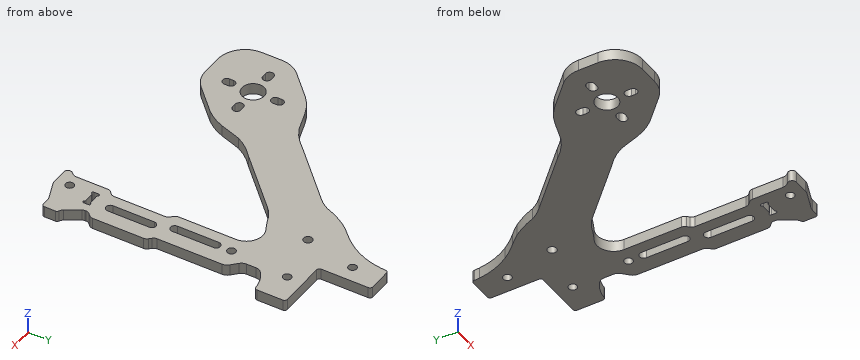
from build123d import *

# Parameters (mm, degrees)
F0_R     = 4
F0_R_2   = 1.5
F0_R_3   = 1.6
F1_DEPTH = 4


# Not quite as in the source:
# - ends of sketch curves that miss each other by under 0.0002 mm in the source are joined


with BuildPart() as f1:
    # F0 (on Top) → F1 (new body)
    with BuildSketch(Plane.XY):
        with BuildLine():
            ThreePointArc((30.9978440056, -52.3819660063), (30.5965854602, -54.0352331312), (31.997844, -55))
            Line((31.997844, -55), (37.420097, -55))
            ThreePointArc((37.420097, -55), (37.9874195635, -54.9458691602), (38.5342690291, -54.7854300727))
            Line((38.5342690291, -54.7854300727), (44.961419, -52.21457))
            ThreePointArc((44.961419, -52.21457), (45.5082684365, -52.0541308398), (46.075591, -52))
            Line((46.075591, -52), (48.497844, -52))
            ThreePointArc((48.497844, -52), (49.2049507812, -51.7071067812), (49.497844, -51))
            Line((49.497844, -51), (49.497844, -47.054858))
            ThreePointArc((49.497844, -47.054858), (49.3143367471, -46.477502309), (48.8311648121, -46.1120445316))
            ThreePointArc((48.8311648121, -46.1120445316), (48.2464480359, -45.7865652768), (47.8018474974, -45.2864046891))
            Line((47.8018474974, -45.2864046891), (44.801847, -40.486405))
            ThreePointArc((44.801847, -40.486405), (44.5753463762, -39.9777725676), (44.497844, -39.426408))
            Line((44.497844, -39.426408), (44.497844, -39.145707))
            ThreePointArc((44.497844, -39.145707), (44.650084935, -38.3803401353), (45.0836304376, -37.7314934376))
            Line((45.0836304376, -37.7314934376), (45.912058, -36.903066))
            ThreePointArc((45.912058, -36.903066), (46.3456032003, -36.2542195381), (46.497844, -35.488853))
            Line((46.497844, -35.488853), (46.497844, -17.145707))
            ThreePointArc((46.497844, -17.145707), (46.345603065, -16.3803401353), (45.9120575624, -15.7314934376))
            Line((45.9120575624, -15.7314934376), (45.08363, -14.903066))
            ThreePointArc((45.08363, -14.903066), (44.6500847997, -14.2542195381), (44.497844, -13.488853))
            Line((44.497844, -13.488853), (44.497844, 9.963987))
            ThreePointArc((44.497844, 9.963987), (44.2491834617, 11.1598679166), (43.5444232222, 12.1575032382))
            Line((43.5444232222, 12.1575032382), (41.451265, 14.110446))
            ThreePointArc((41.451265, 14.110446), (40.7465046743, 15.1080817706), (40.497844, 16.303963))
            Line((40.497844, 16.303963), (40.497844, 19.657184))
            ThreePointArc((40.497844, 19.657184), (40.8005276064, 20.970380205), (41.6475001819, 22.0185877679))
            ThreePointArc((41.6475001819, 22.0185877679), (44.9097367641, 23.8722057946), (48.5706879935, 24.6941080891))
            ThreePointArc((48.5706879935, 24.6941080891), (49.2302523646, 25.0105853837), (49.497844, 25.691451))
            Line((49.497844, 25.691451), (49.497844, 35))
            ThreePointArc((49.497844, 35), (49.2049507812, 35.7071067812), (48.497844, 36))
            Line((48.497844, 36), (31.497844, 36))
            ThreePointArc((31.497844, 36), (30.7907372188, 36.2928932188), (30.497844, 37))
            Line((30.497844, 37), (30.497844, 54))
            ThreePointArc((30.497844, 54), (30.2049507812, 54.7071067812), (29.497844, 55))
            Line((29.497844, 55), (21.513528, 55))
            ThreePointArc((21.513528, 55), (20.8178624993, 54.7183658616), (20.5140433064, 54.0320990223))
            ThreePointArc((20.5140433064, 54.0320990223), (20.4696724232, 53.1001685974), (20.3964907955, 52.1700570193))
            ThreePointArc((20.3964907955, 52.1700570193), (19.0508324444, 46.0085107955), (16.2674640132, 40.3491549914))
            ThreePointArc((16.2674640132, 40.3491549914), (14.1457607442, 37.4387671742), (11.7343381171, 34.7635058829))
            ThreePointArc((11.7343381171, 34.7635058829), (10.1184707238, 33.0449295675), (8.6114374257, 31.2301616681))
            ThreePointArc((8.6114374257, 31.2301616681), (6.2460068014, 27.2541578949), (4.4197862212, 23.0034182758))
            ThreePointArc((4.4197862212, 23.0034182758), (3.0950438794, 20.8390250787), (1.4145833361, 18.9375536462))
            Line((1.4145833361, 18.9375536462), (-16.61664, 0.906331))
            ThreePointArc((-16.61664, 0.906331), (-19.8548943434, -2.2936956172), (-23.6877079435, -4.7505231125))
            Line((-23.6877079435, -4.7505231125), (-31.112329, -7.225397))
            ThreePointArc((-31.112329, -7.225397), (-34.8708228196, -8.9751171402), (-38.1833968947, -11.4680371131))
            Line((-38.1833968947, -11.4680371131), (-46.668678, -19.953319))
            ThreePointArc((-46.668678, -19.953319), (-48.7861533831, -23.2075482546), (-49.4971053712, -27.0243870045))
            Line((-49.4971053712, -27.0243870045), (-49.497105, -34.095454))
            ThreePointArc((-49.497105, -34.095454), (-46.5976100448, -41.0954540448), (-39.59761, -43.994949))
            Line((-39.59761, -43.994949), (-32.526543, -43.994949))
            ThreePointArc((-32.526543, -43.994949), (-28.7097042546, -43.2839973831), (-25.455474662, -41.1665223463))
            Line((-25.455474662, -41.1665223463), (-16.970193, -32.681241))
            ThreePointArc((-16.970193, -32.681241), (-14.4772731402, -29.3686668196), (-12.7275523092, -25.6101732374))
            Line((-12.7275523092, -25.6101732374), (-10.252679, -18.185552))
            ThreePointArc((-10.252679, -18.185552), (-7.7958516172, -14.3527383434), (-4.5958249273, -11.1144840887))
            Line((-4.5958249273, -11.1144840887), (13.497844, 7))
            ThreePointArc((13.497844, 7), (15.3717346163, 8.6360982299), (17.5012621548, 9.9219426844))
            ThreePointArc((17.5012621548, 9.9219426844), (20.331733184, 11.063946628), (23.0532060982, 12.4457298257))
            ThreePointArc((23.0532060982, 12.4457298257), (29.0253982797, 12.3981522415), (31.997844, 7.218006))
            Line((31.997844, 7.218006), (31.997844, -13.488853))
            ThreePointArc((31.997844, -13.488853), (32.1500847997, -14.2542195381), (32.5836299376, -14.9030660624))
            Line((32.5836299376, -14.9030660624), (33.412058, -15.731493))
            ThreePointArc((33.412058, -15.731493), (33.845603065, -16.3803401353), (33.997844, -17.145707))
            Line((33.997844, -17.145707), (33.997844, -35.488853))
            ThreePointArc((33.997844, -35.488853), (33.8456032003, -36.2542195381), (33.4120580624, -36.9030660624))
            Line((33.4120580624, -36.9030660624), (32.58363, -37.731493))
            ThreePointArc((32.58363, -37.731493), (32.150084935, -38.3803401353), (31.997844, -39.145707))
            Line((31.997844, -39.145707), (31.997844, -50.145898))
            ThreePointArc((31.997844, -50.145898), (31.7364567845, -51.3706428782), (30.9978440056, -52.3819660063))
        make_face()
        with BuildLine():
            ThreePointArc((-33.319436, -34.31728), (-31.819436, -32.81728), (-30.319436, -34.31728))
            Line((-30.319436, -34.31728), (-30.319436, -35.81728))
            ThreePointArc((-30.319436, -35.81728), (-31.819436, -37.31728), (-33.319436, -35.81728))
            Line((-33.319436, -35.81728), (-33.319436, -34.31728))
        make_face(mode=Mode.SUBTRACT)
        with BuildLine():
            ThreePointArc((-41.319436, -27.81728), (-42.819436, -26.31728), (-41.319436, -24.81728))
            Line((-41.319436, -24.81728), (-39.819436, -24.81728))
            ThreePointArc((-39.819436, -24.81728), (-38.319436, -26.31728), (-39.819436, -27.81728))
            Line((-39.819436, -27.81728), (-41.319436, -27.81728))
        make_face(mode=Mode.SUBTRACT)
        with Locations((-31.819436, -26.31728)):
            Circle(F0_R, mode=Mode.SUBTRACT)
        with BuildLine():
            ThreePointArc((-33.319436, -16.81728), (-31.819436, -15.31728), (-30.319436, -16.81728))
            Line((-30.319436, -16.81728), (-30.319436, -18.31728))
            ThreePointArc((-30.319436, -18.31728), (-31.819436, -19.81728), (-33.319436, -18.31728))
            Line((-33.319436, -18.31728), (-33.319436, -16.81728))
        make_face(mode=Mode.SUBTRACT)
        with BuildLine():
            ThreePointArc((-23.819436, -27.81728), (-25.319436, -26.31728), (-23.819436, -24.81728))
            Line((-23.819436, -24.81728), (-22.319436, -24.81728))
            ThreePointArc((-22.319436, -24.81728), (-20.819436, -26.31728), (-22.319436, -27.81728))
            Line((-22.319436, -27.81728), (-23.819436, -27.81728))
        make_face(mode=Mode.SUBTRACT)
        with Locations((36.497844, -50)):
            Circle(F0_R_2, mode=Mode.SUBTRACT)
        with BuildLine():
            Line((41.522844, -40.125), (41.522844, -41.875))
            ThreePointArc((41.522844, -41.875), (41.1522534506, -42.3579629324), (40.5898312236, -42.1249998709))
            ThreePointArc((40.5898312236, -42.1249998709), (40.406818848, -41.9419872104), (40.156819, -41.875))
            Line((40.156819, -41.875), (36.838869, -41.875))
            ThreePointArc((36.838869, -41.875), (36.588869152, -41.9419872104), (36.4058564736, -42.1249996961))
            ThreePointArc((36.4058564736, -42.1249996961), (35.8434345494, -42.3579629324), (35.472844, -41.875))
            Line((35.472844, -41.875), (35.472844, -40.125))
            ThreePointArc((35.472844, -40.125), (35.8434345494, -39.6420370676), (36.4058567764, -39.8750001291))
            ThreePointArc((36.4058567764, -39.8750001291), (36.588869152, -40.0580127896), (36.838869, -40.125))
            Line((36.838869, -40.125), (40.156819, -40.125))
            ThreePointArc((40.156819, -40.125), (40.406818848, -40.0580127896), (40.5898315264, -39.8750003039))
            ThreePointArc((40.5898315264, -39.8750003039), (41.1522534506, -39.6420370676), (41.522844, -40.125))
        make_face(mode=Mode.SUBTRACT)
        with BuildLine():
            Line((40.997844, -18.5), (40.997844, -33.5))
            ThreePointArc((40.997844, -33.5), (39.497844, -35), (37.997844, -33.5))
            Line((37.997844, -33.5), (37.997844, -18.5))
            ThreePointArc((37.997844, -18.5), (39.497844, -17), (40.997844, -18.5))
        make_face(mode=Mode.SUBTRACT)
        with BuildLine():
            Line((38.997844, 3.5), (38.997844, -11.5))
            ThreePointArc((38.997844, -11.5), (37.497844, -13), (35.997844, -11.5))
            Line((35.997844, -11.5), (35.997844, 3.5))
            ThreePointArc((35.997844, 3.5), (37.497844, 5), (38.997844, 3.5))
        make_face(mode=Mode.SUBTRACT)
        with Locations((20.497844, 26)):
            Circle(F0_R_3, mode=Mode.SUBTRACT)
        with Locations((37.497844, 9)):
            Circle(F0_R_2, mode=Mode.SUBTRACT)
        with Locations((24.673148, 44.716341)):
            Circle(F0_R_2, mode=Mode.SUBTRACT)
        with Locations((39.215118, 30.174371)):
            Circle(F0_R_2, mode=Mode.SUBTRACT)
    extrude(amount=F1_DEPTH)


solid = f1.part
Here's how the part is built. I have some questions about the finished solid (model axes, mm). Round coordinates to 2 decimals unless told otherwise and drop trailing zeros. Loops run counter-clockwise (first coordinate to the right, second up) from the corner with the lowest first, then second, coordinate; pieces in that order, holes last. Notation, with made-up numbers: (51.5, 25.5) - (88.5, 25.5) arc R28 ccw to (88.5, 55.5) - close; hole circle Ø2 at (-35, 49.25). An arc over 180 degrees is marked (long way). One line per question, with ' | ' between items. Start each with the question number.
Q1. I want a section at C-C (z = 0.75). State how many separate pieces and enclosed holes the cut face has, then the cut area to 3 significant figures.
Q2. Please list where these lines run through material, in increasing order: line 1 (X direction, y = 4.5, z = 3.2); line 2 (X direction, y = 1.5, z = 1.1); line 3 (X direction, y = -29, z = 0.55). Write a range as [from, to].
Q3. I want a section at B-B (y = 42). Write out the boundary of the cut face in (x, z).
Q4. Will these pins go through, and if not, where does the flat tip stop? pin 1 (1.2 mm diameter, centred on y = -18, z = 1.5, fed in from +X); pin 2 (1.2 mm diameter, centred on x = 47.5, z = 1.5, fed in from -Y).
Q5. I want a section at A-A (x = -2). Write out the boundary of the cut face in (y, z), then the cut area to 3 significant figures.
Response values:
1) separate pieces: 1 | enclosed holes: 13 | area: 3,480 mm²
2) line 1: x = [-13.02, 11], [32, 36.38], [38.62, 44.5] | line 2: x = [-16.02, 8], [32, 36], [39, 44.5] | line 3: x = [-49.5, -34.79], [-28.85, -14.26], [34, 38], [41, 46.5]
3) outline: (17.26, 0) - (30.5, 0) - (30.5, 4) - (17.26, 4) - close
4) pin 1: stops at x = 46.5 | pin 2: stops at y = -52
5) outline: (-8.52, 0) - (15.52, 0) - (15.52, 4) - (-8.52, 4) - close | area: 96.2 mm²
